Autodesk Inventor part; units mm, degrees
ref_plane "Work Plane4" through (0, 5, 0) normal (0, 1, 0) x (1, 0, 0)
ref_plane "YZ Plane" through (0, 0, 0) normal (1, 0, 0) x (0, 1, 0)
ref_plane "XZ Plane" through (0, 0, 0) normal (0, 1, 0) x (-1, 0, 0)
sketch "Sketch1" plane through (0, 0, 0) normal (0, 1, 0) x (-1, 0, 0)
  line L0 (30, 30) -> (-30, 30)
  line L1 (-30, 30) -> (-30, -30)
  line L2 (-30, -30) -> (30, -30)
  line L3 (30, -30) -> (30, 30)
  line L4 (30, 30) -> (-30, -30) construction
  line L5 (-30, 30) -> (30, -30) construction
  point P0 (0, 0)
  dimension "d0" = 60
  dimension "d1" = 60
extrude "Extrusion1" add sketch "Sketch1" along normal blind 10
fillet "Fillet1" radius 7 4 edges at (30, 5, 30) (30, 5, -30) (-30, 5, 30) (-30, 5, -30)
sketch "Sketch2" plane through (0, 10, 0) normal (0, 1, 0) x (1, 0, 0)
  line L0 (-30, 30) -> (30, 30)
  line L1 (30, 30) -> (30, -30)
  line L2 (30, -30) -> (-30, -30)
  line L3 (-30, -30) -> (-30, 30)
  line L4 (-30, 30) -> (30, -30) construction
  line L5 (30, 30) -> (-30, -30) construction
  line L6 (25, -25) -> (25, 25)
  line L7 (25, 25) -> (-25, 25)
  line L8 (-25, 25) -> (-25, -25)
  line L9 (-25, -25) -> (25, -25)
  circle A0 centre (25, -25) radius 2.75
  circle A1 centre (-25, -25) radius 2.75
  circle A2 centre (25, 25) radius 2.75
  circle A3 centre (-25, 25) radius 2.75
  point P0 (0, 0)
  dimension "d5" = 5
  dimension "d6" = 5.5
  dimension "d7" = 5.5
  dimension "d8" = 5.5
  dimension "d9" = 5.5
extrude "Extrusion2" cut sketch "Sketch2" against normal blind 3 contours L9 A0 L6 | L6 A0 L9 | A2 L7 L6 | L6 L7 A2 | A1 L8 L9 | L9 L8 A1 | A3 L8 L7 | L7 L8 A3
sketch "Sketch7" plane through (0, 10, 0) normal (0, 1, 0) x (1, 0, 0)
  line L0 (-23, 30) -> (23, 30)
  line L1 (30, 23) -> (30, -23)
  line L2 (23, -30) -> (-23, -30)
  line L3 (-30, -23) -> (-30, 23)
  line L4 (-30, 30) -> (30, -30) construction
  line L5 (30, 30) -> (-30, -30) construction
  arc A0 (-23, 30) -> (-30, 23) centre (-23, 23) ccw
  arc A1 (-30, -23) -> (-23, -30) centre (-23, -23) ccw
  arc A2 (23, -30) -> (30, -23) centre (23, -23) ccw
  arc A3 (30, 23) -> (23, 30) centre (23, 23) ccw
  line L6 (23, 32) -> (-23, 32)
  arc A4 (-23, 32) -> (-32, 23) centre (-23, 23) ccw
  line L7 (-32, 23) -> (-32, -23)
  arc A5 (-32, -23) -> (-23, -32) centre (-23, -23) ccw
  line L8 (-23, -32) -> (23, -32)
  arc A6 (23, -32) -> (32, -23) centre (23, -23) ccw
  line L9 (32, -23) -> (32, 23)
  arc A7 (32, 23) -> (23, 32) centre (23, 23) ccw
  point P0 (0, 0)
  dimension "d47" = 7
  dimension "d48" = 2
extrude "Extrusion6" add sketch "Sketch7" against normal blind 10
sketch "Sketch17" plane through (0, 10, 0) normal (0, 1, 0) x (1, 0, 0)
  circle A0 centre (25, -25) radius 2.75
  line L0 (-25, 25) -> (25, 25)
  line L1 (25, 25) -> (25, -25)
  line L2 (25, -25) -> (-25, -25)
  line L3 (-25, -25) -> (-25, 25)
  line L4 (-25, 25) -> (25, -25) construction
  line L5 (25, 25) -> (-25, -25) construction
  line L6 (21, -21) -> (21, 10.7)
  line L7 (-21.4, -13) -> (21, -13)
  line L8 (21, 10.7) -> (-21.4, 10.7)
  line L9 (-21.4, -13) -> (-21.4, 10.7)
  line L10 (-19.4, 9.7) -> (-19.4, -11)
  line L11 (-19.4, -11) -> (19, -11)
  line L12 (19, 9.7) -> (-19.4, 9.7)
  line L13 (19, 9.7) -> (19, -11)
  point P0 (0, 0)
  dimension "d134" = 50
  dimension "d135" = 50
  dimension "d136" = 4
  dimension "d137" = 8
  dimension "d138" = 42.4
  dimension "d139" = 23.7
  dimension "d141" = 1
  dimension "d142" = 2
extrude "Extrusion15" cut sketch "Sketch17" against normal blind 2 contours L7 L9 L8 L6
sketch "Sketch18" plane through (0, 10, 0) normal (0, 1, 0) x (1, 0, 0)
  line L0 (-19.4, 9.7) -> (19, 9.7)
  line L1 (19, 9.7) -> (19, -11)
  line L2 (19, -11) -> (-19.4, -11)
  line L3 (-19.4, -11) -> (-19.4, 9.7)
  point P0 (0, 0)
extrude "Extrusion16" cut sketch "Sketch18" against normal blind 8
sketch "Sketch19" plane through (0, 10, 0) normal (0, 1, 0) x (1, 0, 0)
  line L0 (23, 32) -> (-23, 32)
  line L1 (-32, 23) -> (-32, -23)
  line L2 (32, -23) -> (32, 23)
  line L3 (-21.4, 10.7) -> (21, 10.7)
  line L4 (-18, 14.7) -> (-18, 28)
  line L5 (-18, 28) -> (18, 28)
  line L6 (18, 28) -> (18, 14.7)
  line L7 (18, 14.7) -> (-18, 14.7)
  line L8 (-23, -32) -> (23, -32)
  line L9 (-28, -18) -> (-28, 18)
  line L10 (-21.4, -13) -> (-21.4, 10.7)
  line L11 (-28, -18) -> (-25.4, -18)
  line L12 (-25.4, -18) -> (-25.4, 18)
  line L13 (-25.4, 18) -> (-28, 18)
  line L14 (21, 10.7) -> (21, -13)
  line L15 (28, 18) -> (25, 18)
  line L16 (25, 18) -> (25, -18)
  line L17 (25, -18) -> (28, -18)
  line L18 (28, -18) -> (28, 18)
  line L19 (21, -13) -> (-21.4, -13)
  line L20 (18, -28) -> (18, -17)
  line L21 (18, -28) -> (-18, -28)
  line L22 (-18, -28) -> (-18, -17)
  line L23 (-18, -17) -> (18, -17)
  point P0 (0, 0)
  dimension "d147" = 4
  dimension "d148" = 14
  dimension "d149" = 4
  dimension "d150" = 14
  dimension "d151" = 4
  dimension "d152" = 4
  dimension "d153" = 4
  dimension "d154" = 4
  dimension "d155" = 14
  dimension "d156" = 14
  dimension "d157" = 4
  dimension "d158" = 4
  dimension "d159" = 14
  dimension "d160" = 4
  dimension "d161" = 14
  dimension "d162" = 4
  dimension "d163" = 4
  dimension "d164" = 4
  dimension "d165" = 14
  dimension "d166" = 14
  dimension "d167" = 4
extrude "Extrusion17" cut sketch "Sketch19" against normal through all contours L4 L5 L6 L7 | L9 L13 L12 L11 | L18 L17 L16 L15 | L21 L22 L23 L20
fillet "Fillet5" radius 2 8 edges at (18, 5, -28) (18, 5, 17) (-18, 5, -28) (-18, 5, 17) (-18, 5, -14.7) (-18, 5, 28) (18, 5, -14.7) (18, 5, 28)
fillet "Fillet5" radius 0.5 12 edges at (28, 5, 18) (-25.4, 5, 18) (28, 5, -18) (-25.4, 5, -18) (-28, 5, -18) (25, 5, -18) (-0.2, 2, -9.7) (-19.4, 2, 0.65) (-0.2, 2, 11) (-28, 5, 18) (25, 5, 18) (19, 2, 0.65)
ref_plane "Work Plane4" through (0, 5, 0) normal (0, 1, 0) x (1, 0, 0)
mirror "Mirror4" about plane through (0, 5, 0) normal (0, 1, 0) of "Extrusion2"
properties part number "14 pin long holder"
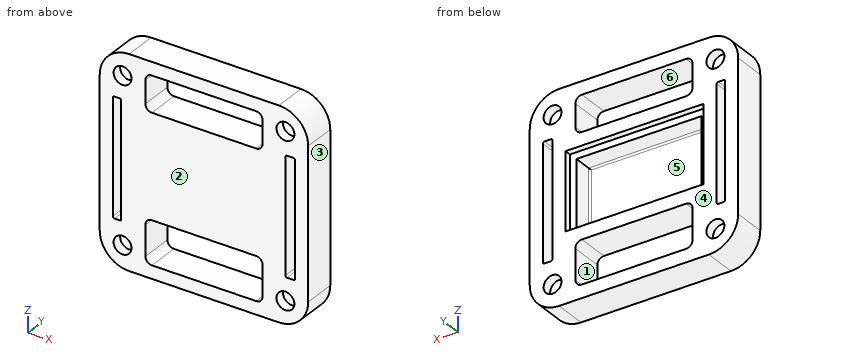
Work out the finished part from the listing and answer in its coordinate system (mm). Face numbers are marked on the shaded views. A direction names the side the tool comes from. Round coordinates to 2 decimals unless told otherwise and drop trailing zeros. Order: outer loops, then holes, each group sorted by start corner. A loop starts at its lowest first (then second) coordinate and runs counter-clockwise, first axis right, second up. Notation, with made-up numbers: M -2,62.5 L 4,62.5 A12 cw 4,70.5 Z; hole C -27,82.25 d7. An arc over 180 degrees is marked long. Put each result on its own line as item: value. Start each with the question number.
Q1. A tool of negligible diameter and unlimited length cuts with its end or side. For the marked faces 4, 5 and 6, from which of +Z, -Z, +X, -X, +Y, -Y can it reach the whole face along a straight path? Write none if from no direction.
Q2. Straight lines are drawn through the part: L1, parallel to Z at x = 1, y = 1.25; L2, parallel to Z at x = 11, y = 5.75; L3, parallel to X at y = 8.5, z = -11. For each, find the intervals that lie inside material, in ascending order. Write a range as [from, to].
Q3. For a pull along X with two mould halves and no side action, classify the marked faces 1, 2 and 3 as pulls with the +X half, pulls with the -X half, needs draft (parallel to the pull), parting line crosses it, or undercut.
Q4. Flat-ended cylindrical pins translate along their axes: pin 1 (0.8 mm diameter, centred on x = -27, y = 3, fed in from +Z); pin 2 (5 mm diameter, centred on x = 25, z = -25, fed in from -Y); pin 3 (3 mm diameter, centred on x = 25, z = 24.5, fed in from +Y). Find the tip coordinate at first contact, or state that the pin passes through.
Q5. Section C-C, the plane z = 25 is taken. Write down the section's boundary in (x, y).
Q6. Section A-A, the plane x = 4 is taken. Write down the section's boundary in (y, z), and give its area (3 significant figures).
Q7. Section B-B, the plane z = 5 is taken. Write down the section's boundary in (x, y), and give its area (3 significant figures).
Findings below:
1. face 4: +Z, -Z, +X, -X, +Y
1. face 5: +Y
1. face 6: +Y, -Y
2. L1: z = [-32, -28], [-14.7, 17], [28, 32]
2. L2: z = [-32, -28], [-14.7, -9.7], [11, 17], [28, 32]
2. L3: x = [-32, -28], [-25.4, 25], [28, 32]
3. face 1: undercut
3. face 2: needs draft
3. face 3: pulls with the +X half
4. pin 1: stops at z = 31.25
4. pin 2: stops at y = 3
4. pin 3: stops at y = 7
5. outline: M -31.77,0 L -27.75,0 L -27.75,3 L -22.25,3 L -22.25,0 L -18,0 L -18,10 L -22.25,10 L -22.25,7 L -27.75,7 L -27.75,10 L -31.77,10 Z; M 18,0 L 22.25,0 L 22.25,3 L 27.75,3 L 27.75,0 L 31.77,0 L 31.77,10 L 27.75,10 L 27.75,7 L 22.25,7 L 22.25,10 L 18,10 Z
6. outline: M 0,-32 L 10,-32 L 10,-28 L 0,-28 Z; M 0,-14.7 L 10,-14.7 L 10,-10.7 L 8,-10.7 L 8,-9.7 L 2.5,-9.7 A0.5 cw 2,-9.2 L 2,10.5 A0.5 cw 2.5,11 L 8,11 L 8,13 L 10,13 L 10,17 L 0,17 Z; M 0,28 L 10,28 L 10,32 L 0,32 Z
6. area: 226 mm^2
7. outline: M -32,0 L -28,0 L -28,10 L -32,10 Z; M -25.4,0 L 25,0 L 25,10 L 21,10 L 21,8 L 19,8 L 19,2.5 A0.5 cw 18.5,2 L -18.9,2 A0.5 cw -19.4,2.5 L -19.4,8 L -21.4,8 L -21.4,10 L -25.4,10 Z; M 28,0 L 32,0 L 32,10 L 28,10 Z
7. area: 269 mm^2
